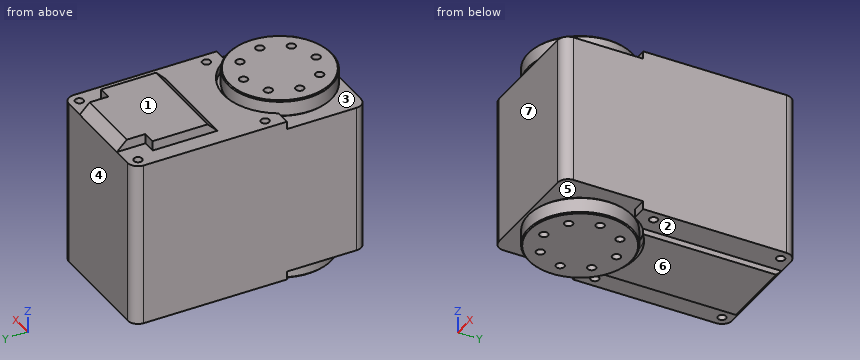
from build123d import *

# Parameters (mm, degrees)
BOSS_EXTRUDE1_DEPTH      = 32
CUT_EXTRUDE1_START       = -1.5
CUT_EXTRUDE1_DEPTH       = 1.5
SKETCH3_R                = 10.8
SKETCH3_W                = 24.5
SKETCH3_H                = 15.4
CUT_EXTRUDE2_DEPTH       = 1.6
BOSS_EXTRUDE2_DEPTH      = 0.3
BOSS_EXTRUDE2_DEPTH_BACK = 29.3
SKETCH4_R                = 3.2
SKETCH5_R                = 10
SKETCH5_R_2              = 0.8
BOSS_EXTRUDE3_DEPTH      = 3.2
BOSS_EXTRUDE5_START      = 3.2
SKETCH6_R                = 10
SKETCH6_R_2              = 0.8
BOSS_EXTRUDE5_DEPTH      = 3.2
BOSS_EXTRUDE6_DEPTH      = 1.9
CHAMFER1_SIZE            = 1.9
BOSS_EXTRUDE7_START      = 1.1
BOSS_EXTRUDE7_DEPTH      = 1.1
CHAMFER2_SIZE            = 1.1
SKETCH9_R                = 0.8
CUT_EXTRUDE3_DEPTH       = 3
CUT_EXTRUDE4_START       = -3
SKETCH10_R               = 0.8
CUT_EXTRUDE4_DEPTH       = 3
CHAMFER3_SIZE            = 0.2


with BuildPart() as part:
    # Sketch1 → Boss-Extrude1 (new body)
    with BuildSketch(Plane.XY):
        with BuildLine():
            Line((-10.25, 22.5), (10.25, 22.5))
            ThreePointArc((10.25, 22.5), (11.664213562, 21.914213562), (12.25, 20.5))
            Line((12.25, 20.5), (12.25, -20.5))
            ThreePointArc((12.25, -20.5), (11.664213562, -21.914213562), (10.25, -22.5))
            Line((10.25, -22.5), (-10.25, -22.5))
            ThreePointArc((-10.25, -22.5), (-11.664213562, -21.914213562), (-12.25, -20.5))
            Line((-12.25, -20.5), (-12.25, 20.5))
            ThreePointArc((-12.25, 20.5), (-11.664213562, 21.914213562), (-10.25, 22.5))
        make_face()
    extrude(amount=BOSS_EXTRUDE1_DEPTH)

    # Sketch2 → Cut-Extrude1 (cut)
    with BuildSketch(Plane.XY.offset(32).offset(CUT_EXTRUDE1_START)):
        with BuildLine():
            ThreePointArc((9.353074361, -7.1), (0, -1.7), (-9.353074361, -7.1))
            Line((-9.353074361, -7.1), (9.353074361, -7.1))
        make_face()
        with BuildLine():
            Line((9.353074361, -7.1), (-9.353074361, -7.1))
            ThreePointArc((-9.353074361, -7.1), (-10.217465609, -15.99905652), (-4.079215611, -22.5))
            Line((-4.079215611, -22.5), (4.079215611, -22.5))
            ThreePointArc((4.079215611, -22.5), (8.963691444, -18.524303752), (10.8, -12.5))
            ThreePointArc((10.8, -12.5), (10.431998924, -9.704754313), (9.353074361, -7.1))
        make_face()
        with BuildLine():
            Line((12.25, -7.1), (9.353074361, -7.1))
            ThreePointArc((9.353074361, -7.1), (10.431998924, -9.704754313), (10.8, -12.5))
            ThreePointArc((10.8, -12.5), (8.963691444, -18.524303752), (4.079215611, -22.5))
            Line((4.079215611, -22.5), (10.25, -22.5))
            ThreePointArc((10.25, -22.5), (11.664213562, -21.914213562), (12.25, -20.5))
            Line((12.25, -20.5), (12.25, -7.1))
        make_face()
        with BuildLine():
            Line((-9.353074361, -7.1), (-12.25, -7.1))
            Line((-12.25, -7.1), (-12.25, -20.5))
            ThreePointArc((-12.25, -20.5), (-11.664213562, -21.914213562), (-10.25, -22.5))
            Line((-10.25, -22.5), (-4.079215611, -22.5))
            ThreePointArc((-4.079215611, -22.5), (-10.217465609, -15.99905652), (-9.353074361, -7.1))
        make_face()
    extrude(amount=CUT_EXTRUDE1_DEPTH, mode=Mode.SUBTRACT)

    # Sketch3 → Cut-Extrude2 (cut)
    with BuildSketch(Plane(origin=(0, 0, 0), x_dir=(-1, 0, 0), z_dir=(0, 0, -1))):
        with Locations((0, -12.5)):
            Circle(SKETCH3_R)
        with Locations((0, -14.8)):
            Rectangle(SKETCH3_W, SKETCH3_H)
    extrude(amount=-CUT_EXTRUDE2_DEPTH, mode=Mode.SUBTRACT)

    # Sketch4 → Boss-Extrude2 (add, two sides: drawn at the far end of the back side and taken through both)
    with BuildSketch(Plane.XY.offset(30.5).offset(-BOSS_EXTRUDE2_DEPTH_BACK)):
        with Locations((0, -12.5)):
            Circle(SKETCH4_R)
    extrude(amount=BOSS_EXTRUDE2_DEPTH + BOSS_EXTRUDE2_DEPTH_BACK)

    # Sketch5 → Boss-Extrude3 (add)
    with BuildSketch(Plane.XY.offset(30.8)):
        with Locations((0, -12.5)):
            Circle(SKETCH5_R)
        with Locations((0, -5.5)):
            Circle(SKETCH5_R_2, mode=Mode.SUBTRACT)
        with Locations((4.949747468, -7.550252532)):
            Circle(SKETCH5_R_2, mode=Mode.SUBTRACT)
        with Locations((7, -12.5)):
            Circle(SKETCH5_R_2, mode=Mode.SUBTRACT)
        with Locations((4.949747468, -17.449747468)):
            Circle(SKETCH5_R_2, mode=Mode.SUBTRACT)
        with Locations((0, -19.5)):
            Circle(SKETCH5_R_2, mode=Mode.SUBTRACT)
        with Locations((-4.949747468, -17.449747468)):
            Circle(SKETCH5_R_2, mode=Mode.SUBTRACT)
        with Locations((-7, -12.5)):
            Circle(SKETCH5_R_2, mode=Mode.SUBTRACT)
        with Locations((-4.949747468, -7.550252532)):
            Circle(SKETCH5_R_2, mode=Mode.SUBTRACT)
    extrude(amount=BOSS_EXTRUDE3_DEPTH)

    # Sketch6 → Boss-Extrude5 (add)
    with BuildSketch(Plane(origin=(0, 0, 1.2), x_dir=(-1, 0, 0), z_dir=(0, 0, -1)).offset(BOSS_EXTRUDE5_START)):
        with Locations(Location((0, -12.5, 0), (0, 0, 180))):
            Circle(SKETCH6_R)
        with Locations(Location((0, -5.5, 0), (0, 0, 180))):
            Circle(SKETCH6_R_2, mode=Mode.SUBTRACT)
        with Locations(Location((4.949747468, -7.550252532, 0), (0, 0, 180))):
            Circle(SKETCH6_R_2, mode=Mode.SUBTRACT)
        with Locations(Location((7, -12.5, 0), (0, 0, 180))):
            Circle(SKETCH6_R_2, mode=Mode.SUBTRACT)
        with Locations(Location((4.949747468, -17.449747468, 0), (0, 0, 180))):
            Circle(SKETCH6_R_2, mode=Mode.SUBTRACT)
        with Locations(Location((0, -19.5, 0), (0, 0, 180))):
            Circle(SKETCH6_R_2, mode=Mode.SUBTRACT)
        with Locations(Location((-4.949747468, -17.449747468, 0), (0, 0, 180))):
            Circle(SKETCH6_R_2, mode=Mode.SUBTRACT)
        with Locations(Location((-7, -12.5, 0), (0, 0, 180))):
            Circle(SKETCH6_R_2, mode=Mode.SUBTRACT)
        with Locations(Location((-4.949747468, -7.550252532, 0), (0, 0, 180))):
            Circle(SKETCH6_R_2, mode=Mode.SUBTRACT)
    extrude(amount=-BOSS_EXTRUDE5_DEPTH)

    # Sketch7 → Boss-Extrude6 (add)
    with BuildSketch(Plane.XY.offset(32)):
        Polygon((6.5, 22.5), (-6.5, 22.5), (-6.5, 17), (-9, 17), (-9, 4.5), (9, 4.5), (9, 17), (6.5, 17), align=None)
    extrude(amount=BOSS_EXTRUDE6_DEPTH)

    # Chamfer1
    chamfer1_edges = [part.edges().sort_by_distance(p)[0] for p in [
        (0, 22.5, 33.9),
        (0, 4.5, 33.9),
    ]]
    chamfer(chamfer1_edges, length=CHAMFER1_SIZE - 0.0001)  # a hair under: the kernel refuses the full size

    # Sketch8 → Boss-Extrude7 (add)
    with BuildSketch(Plane(origin=(0, 0, 0), x_dir=(-1, 0, 0), z_dir=(0, 0, -1)).offset(BOSS_EXTRUDE7_START)):
        with BuildLine():
            Line((7, 22.5), (-7, 22.5))
            Line((-7, 22.5), (-7, -4.275645922))
            ThreePointArc((-7, -4.275645922), (0, -1.7), (7, -4.275645922))
            Line((7, -4.275645922), (7, 22.5))
        make_face()
    extrude(amount=-BOSS_EXTRUDE7_DEPTH)

    # Chamfer2
    chamfer2_edges = [part.edges().sort_by_distance(p)[0] for p in [
        (0, 22.5, -1.1),
    ]]
    chamfer(chamfer2_edges, length=CHAMFER2_SIZE)

    # Sketch9 → Cut-Extrude3 (cut)
    with BuildSketch(Plane.XY.offset(32)):
        with Locations((-10.25, 20.5)):
            Circle(SKETCH9_R)
        with Locations((10.25, 20.5)):
            Circle(SKETCH9_R)
        with Locations((-10.25, -4)):
            Circle(SKETCH9_R)
        with Locations((10.25, -4)):
            Circle(SKETCH9_R)
    extrude(amount=-CUT_EXTRUDE3_DEPTH, mode=Mode.SUBTRACT)

    # Sketch10 → Cut-Extrude4 (cut)
    with BuildSketch(Plane(origin=(0, 0, 0), x_dir=(-1, 0, 0), z_dir=(0, 0, -1)).offset(CUT_EXTRUDE4_START)):
        with Locations(Location((-10.25, 20.5, 0), (0, 0, 180))):
            Circle(SKETCH10_R)
        with Locations(Location((10.25, 20.5, 0), (0, 0, 180))):
            Circle(SKETCH10_R)
        with Locations(Location((-10.25, -4, 0), (0, 0, 180))):
            Circle(SKETCH10_R)
        with Locations(Location((10.25, -4, 0), (0, 0, 180))):
            Circle(SKETCH10_R)
    extrude(amount=CUT_EXTRUDE4_DEPTH, mode=Mode.SUBTRACT)

    # Chamfer3
    chamfer3_edges = [part.edges().sort_by_distance(p)[0] for p in [
        (-10, -12.5, -2),
        (-10, -12.5, 1.2),
        (-10, -12.5, 34),
        (-10, -12.5, 30.8),
    ]]
    chamfer(chamfer3_edges, length=CHAMFER3_SIZE)


solid = part.part
The listing builds one solid part. Answer for the finished solid, in the listing's coordinates (mm). Face numbers are marked on the shaded views. A direction names the side the tool comes from. Give positions to 0.01 mm unless a question says otherwise; leave off trailing zeros. Write each loop counter-clockwise with the first axis right and the second up, starting at its lowest first coordinate (ties: lowest second). Pieces come first, ordered by that corner, then holes. Notation, with made-up numbers: (33, 51) - (38, 51) arc R31 cw to (38, 79) - close; hole circle Ø10 at (-11, 78.25). An arc over 180 degrees is marked (long way). Use a Markdown table: item, result.
1. For a pull along Y with two mould halves and no side action, classify the marked faces 4, 5, 6 and 7 as released by +Y, released by -Y, zero draft, split by the parting line, or undercut.
Values follow:
| item | result |
|---|---|
| face 4 | released by +Y |
| face 5 | undercut |
| face 6 | zero draft |
| face 7 | released by -Y |
2. Section A-A on y = 2 is taken. Write down the section's boundary in (x, z).
Values follow:
| item | result |
|---|---|
| outline | (-12.25, 0) - (-7, 0) - (-7, -1.1) - (7, -1.1) - (7, 0) - (12.25, 0) - (12.25, 32) - (-12.25, 32) - close |
3. A tool of negligible diameter and unlimited length cuts with its end or side. For the marked faces 1, 2 and 3, from which of +Z, -Z, +X, -X, +Y, -Y can it reach the whole face along a straight path? Write none if from no direction.
Values follow:
| item | result |
|---|---|
| face 1 | +Z, +X, -X, +Y |
| face 2 | -Z, +X, +Y |
| face 3 | none |
4. Find the intervals of material crossed by probe 1 along Y at (x, z) = (-10.25, 2.05); probe 2 along Y at (x, z) = (-10.25, 0.9); probe 3 along Z at (x, y) = (-0.5, -8.5), in increasing order. Write a range as from..to.
Values follow:
| item | result |
|---|---|
| probe 1 | y = -22.5..-4.8, -3.2..19.7, 21.3..22.5 |
| probe 2 | y = -7.1..-4.8, -3.2..19.7, 21.3..22.5 |
| probe 3 | z = -2..1.2, 1.6..30.5, 30.8..34 |
5. Section B-B on x = 0 is taken. Count the separate pieces of the cut face and the enclosed holes in it, plus the area to 3 significant figures.
Values follow:
| item | result |
|---|---|
| separate pieces | 5 |
| enclosed holes | 0 |
| area | 1,540 mm² |
6. Each of these flat-tipped pins is pushed along its axis until it touches: P1, Ø1, axis at x = 4.95, y = -7.55, coming from the +Z side; P2, Ø0.6, axis at y = 13, z = 33, coming from the -X side; P3, Ø1, axis at x = 4.5, y = 3.5, coming from the +Z side. Where does it stop, or does it pass through?
Values follow:
| item | result |
|---|---|
| P1 | stops at z = 30.5 |
| P2 | stops at x = -9 |
| P3 | stops at z = 32 |
